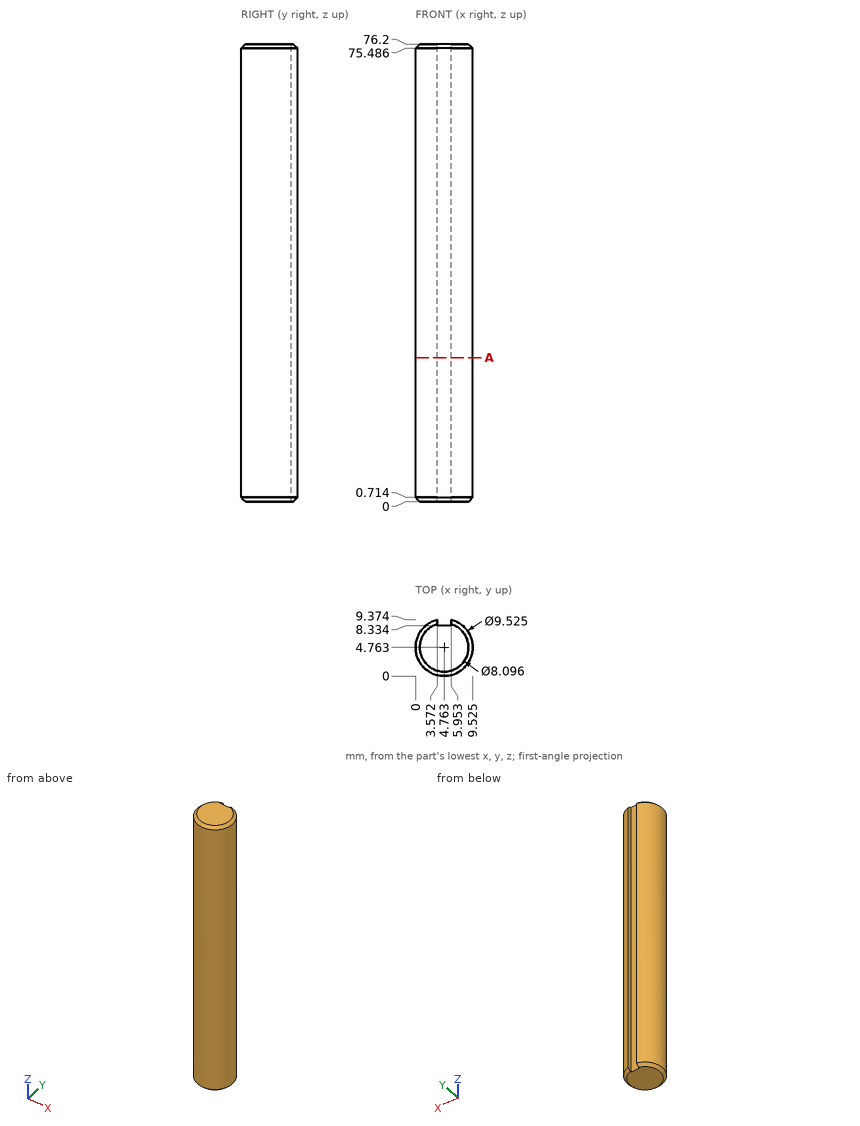
Here's the drawing with two shaded views (mm, measured from the low corner). I have some questions. Coordinates: 2 decimals unless noted, no trailing zeros. Order: outer loops, then holes, each group sorted by start corner. A loop starts at its lowest first (then second) coordinate and runs counter-clockwise, first axis right, second up.
Item 1: If we section it at A-A, the plane z = 24: List the corners of the cut face in (x, y) for me (1 decimal).
Response values:
outline: (3.6, 8.3) - (3.6, 9.4) arc R4.8 ccw (long way) to (6, 9.4) - (6, 8.3) - close
Item 2: I need wall thicknesses on probe 1 along Y at (x, z) = (2.25, 18.5) (1 decimal); probe 2 along X at (y, z) = (5, 48.5) (1 decimal); probe 3 along X at (y, z) = (5.75, 55). Which ranges of each line are inside material? Lowest first, please.
Response values:
probe 1: y = 0.7 to 8.8
probe 2: x = 0 to 9.5
probe 3: x = 0.1 to 9.42
Item 3: I'm going to push flat-ended pins straight in: pin 1 Ø0.5 at (y, z) = (9, 23.5) entering from -X; pin 2 Ø3 at (x, z) = (5, 31.5) entering from +Y; pin 3 Ø1.5 at (y, z) = (2.5, 41) entering from -X; pin 4 Ø0.5 at (y, z) = (9, 53) entering from +X (1 decimal). Where does each tip first touch, or does it pass through?
Response values:
pin 1: stops at x = 2.16
pin 2: stops at y = 9.37
pin 3: stops at x = 0.25
pin 4: stops at x = 7.4
